Could you check a few things on this model? Use its own coordinates, in mm. A direction names the side the tool comes from. Give positions to 0.01 mm unless a question says otherwise; leave off trailing zeros. Loops run counter-clockwise (first coordinate to the right, second up) from the corner with the lowest first, then second, coordinate; pieces in that order, holes last. Notation, with made-up numbers: M 61.25,-28.5 L 103.25,-28.5 A15 cw 103.25,-12.5 Z; hole C 64,80 d5. An arc over 180 degrees is marked long. Use a Markdown table: item, result. Add a question column.
1) Will these pins go through, and if not, where does the flat tip stop? pin 1 Ø23 at (y, z) = (6, -23.5) entering from +X; pin 2 Ø0.8 at (x, y) = (-25, 20) entering from -Z; pin 3 Ø10 at (x, y) = (-49, 26) entering from +Z.
2) Which directions (+Z, -Z, +X, -X, +Y, -Y) give clear straight access to the entire face, cutting with the end or side of a thin tool? Please do faces 5 (the flat face through (-26.149, 8, -22)), 6 (the flat face through (-62.199, 19, 27)), 7 (the flat face through (-27, 19, -22)).
3) We'd pull the mould along Z, two halves only. Please class faces 1 (the flat face through (-24.399, 19, 25)), 2 (the flat face through (-27, 9, -47.607)), 3 (the flat face through (-28.149, 8, -22)), 4 (the flat face through (-62.899, 19, 25)): +Z half, -Z half, draft (parallel to the pull), parting line (faces both ways), or undercut.
4) If I drill on line 1 along X through (y, z) = (11.5, -36); line 2 along X through (y, z) = (28.5, 5.5); line 3 along Z through (x, y) = (-25, 3.5), over which ranges is the centre line in solid material (lowest first)? Write a range as [from, to].
5) Suppose I cut it at B-B on x = -40. List the corners of the cut face in (y, z) for me.
6) Suppose I cut it at D-D on z = 22.5. List the corners of the cut face in (x, y) for me.
7) Suppose I cut it at A-A on z = 7. List the corners of the cut face in (x, y) for me.
8) Suppose I cut it at C-C on y = 34. List the corners of the cut face in (x, z) for me, and give its area (3 significant figures).
```python
from build123d import *

# Parameters (mm, degrees)
BOSS_EXTRUDE1_DEPTH   = 38
BOSS_EXTRUDE1_2_DEPTH = 38
SKETCH2_W             = 42.5
SKETCH2_H             = 5.7
BOSS_EXTRUDE2_DEPTH   = 2
BOSS_EXTRUDE3_DEPTH   = 18
SKETCH4_W             = 42.5
SKETCH4_H             = 40
BOSS_EXTRUDE4_DEPTH   = 2
SKETCH5_W             = 37.1
SKETCH5_H             = 11.85
CUT_EXTRUDE1_DEPTH    = 81.281509747
SKETCH6_W             = 2
SKETCH6_H             = 21
BOSS_EXTRUDE6_DEPTH   = 50


with BuildPart() as part:
    # Sketch1 → Boss-Extrude1 (new body)
    with BuildSketch(Plane(origin=(0, 0, 0), x_dir=(1, 0, 0), z_dir=(0, 1, 0))):
        Polygon((-62.898983402, -26.09346473), (-62.898983402, -24.39346473), (-62.198983402, -24.39346473), (-62.198983402, -22.39346473), (-64.898983402, -22.39346473), (-64.898983402, -28.09346473), (-62.198983402, -28.09346473), (-62.198983402, -26.09346473), align=None)
    extrude(amount=BOSS_EXTRUDE1_DEPTH)



with BuildPart() as body_2:
    # Sketch1 → Boss-Extrude1 2 (new body)
    with BuildSketch(Plane(origin=(0, 0, 0), x_dir=(1, 0, 0), z_dir=(0, 1, 0))):
        Polygon((-25.098983402, -22.39346473), (-25.098983402, -24.39346473), (-24.398983402, -24.39346473), (-24.398983402, -26.09346473), (-25.098983402, -26.09346473), (-25.098983402, -28.09346473), (-22.398983402, -28.09346473), (-22.398983402, -22.39346473), align=None)
    extrude(amount=BOSS_EXTRUDE1_2_DEPTH)


with BuildPart() as part_1:
    add(part.part)

    add(body_2.part)  # Boss-Extrude2 merges body 2
    # Sketch2 → Boss-Extrude2 (add)
    with BuildSketch(Plane(origin=(0, 0, 0), x_dir=(1, 0, 0), z_dir=(0, 1, 0))):
        with Locations((-43.648983402, -25.24346473)):
            Rectangle(SKETCH2_W, SKETCH2_H)
    extrude(amount=-BOSS_EXTRUDE2_DEPTH)

    # Sketch3 → Boss-Extrude3 (add)
    with BuildSketch(Plane(origin=(0, 0, 22.39346473), x_dir=(-1, 0, 0), z_dir=(0, 0, -1))):
        Polygon((64.898983402, 38), (62.198983402, 38), (62.198983402, 0), (25.098983402, 0), (25.098983402, 38), (22.398983402, 38), (22.398983402, -2), (64.898983402, -2), align=None)
    extrude(amount=BOSS_EXTRUDE3_DEPTH)

    # Sketch4 → Boss-Extrude4 (add)
    with BuildSketch(Plane(origin=(0, 0, 4.39346473), x_dir=(-1, 0, 0), z_dir=(0, 0, -1))):
        with Locations((43.648983402, 18)):
            Rectangle(SKETCH4_W, SKETCH4_H)
    extrude(amount=BOSS_EXTRUDE4_DEPTH)

    # Sketch5 → Cut-Extrude1 (cut, through all)
    with BuildSketch(Plane(origin=(0, 0, 0), x_dir=(1, 0, 0), z_dir=(0, 1, 0))):
        with Locations((-43.648983402, -10.31846473)):
            Rectangle(SKETCH5_W, SKETCH5_H)
    extrude(amount=-CUT_EXTRUDE1_DEPTH, mode=Mode.SUBTRACT)

    # Sketch6 → Boss-Extrude6 (add)
    with BuildSketch(Plane(origin=(0, 0, 2.39346473), x_dir=(-1, 0, 0), z_dir=(0, 0, -1))):
        with Locations((27.148983402, 8.5)):
            Rectangle(SKETCH6_W, SKETCH6_H)
        with Locations((60.148983402, 8.5)):
            Rectangle(SKETCH6_W, SKETCH6_H)
    extrude(amount=BOSS_EXTRUDE6_DEPTH)


solid = part_1.part
```
Answer block:
| question | item | result |
|---|---|---|
| 1 | pin 1 | stops at x = -26.15 |
| 1 | pin 2 | stops at z = 2.39 |
| 1 | pin 3 | stops at z = 4.39 |
| 2 | face 5 | -Z, +X, +Y, -Y |
| 2 | face 6 | +Z, +Y |
| 2 | face 7 | -Z, +X, -X, +Y |
| 3 | face 1 | undercut |
| 3 | face 2 | -Z half |
| 3 | face 3 | draft |
| 3 | face 4 | undercut |
| 4 | line 1 | x = [-61.15, -59.15], [-28.15, -26.15] |
| 4 | line 2 | x = [-64.9, -62.2], [-25.1, -22.4] |
| 4 | line 3 | z = [2.39, 24.39], [26.09, 28.09] |
| 5 | outline | M -2,2.39 L 38,2.39 L 38,4.39 L -2,4.39 Z; M -2,16.24 L 0,16.24 L 0,28.09 L -2,28.09 Z |
| 6 | outline | M -64.9,-2 L -22.4,-2 L -22.4,38 L -25.1,38 L -25.1,0 L -62.2,0 L -62.2,38 L -64.9,38 Z |
| 7 | outline | M -64.9,-2 L -62.2,-2 L -62.2,38 L -64.9,38 Z; M -25.1,-2 L -22.4,-2 L -22.4,38 L -25.1,38 Z |
| 8 | outline | M -64.9,2.39 L -22.4,2.39 L -22.4,28.09 L -25.1,28.09 L -25.1,26.09 L -24.4,26.09 L -24.4,24.39 L -25.1,24.39 L -25.1,4.39 L -62.2,4.39 L -62.2,24.39 L -62.9,24.39 L -62.9,26.09 L -62.2,26.09 L -62.2,28.09 L -64.9,28.09 Z |
| 8 | area | 211 mm^2 |
